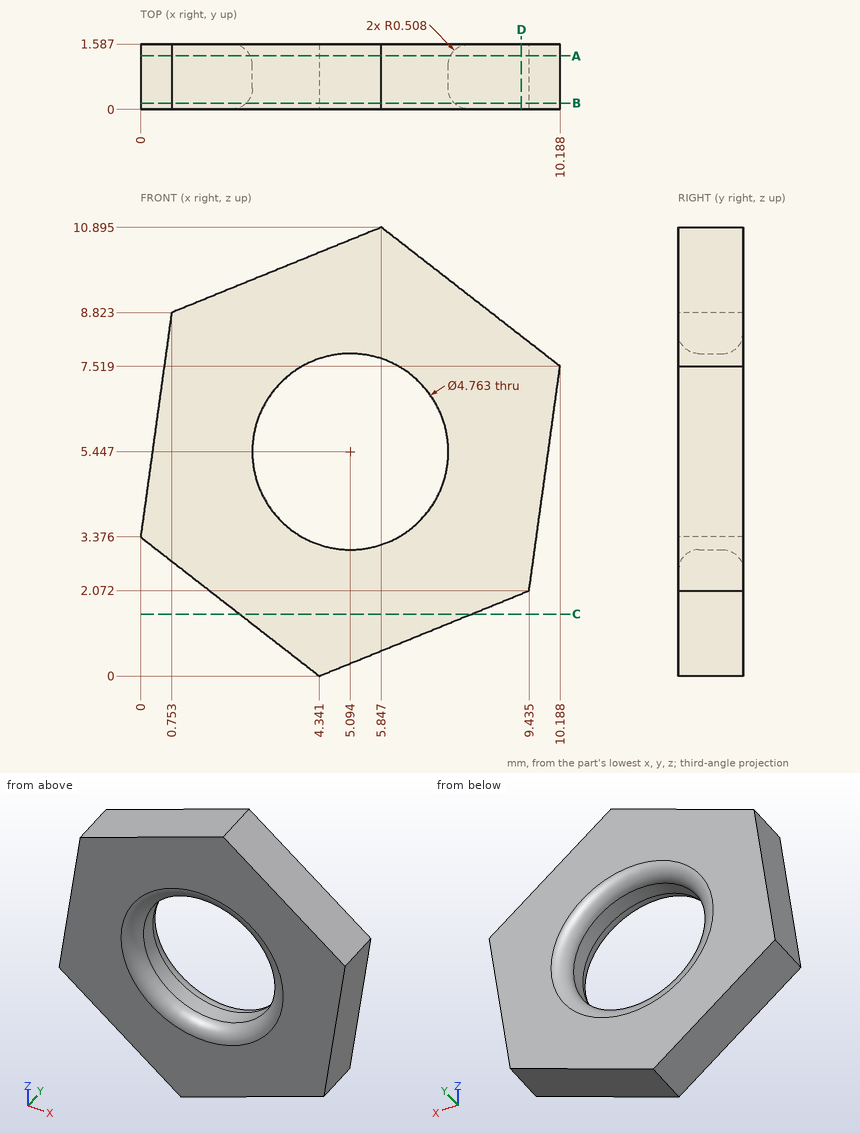
Study the drawing (mm; zero at the part's minimum x, y, z) and answer. Give positions to 0.01 mm unless a question says otherwise; leave off trailing zeros. Loops run counter-clockwise (first coordinate to the right, second up) from the corner with the lowest first, then second, coordinate; pieces in that order, holes last. Notation, with made-up numbers: M -7,-40 L 43,-40 A19 cw 43,-7 Z; hole C 79.25,70.5 d1. An arc over 180 degrees is marked long. Use CSV: the item, a comma, the result in double quotes.
1) Find section B-B on y = 0.15. Write down the section's boundary in (x, z) (1 decimal).
Answer:
outline,"M 0,3.4 L 4.3,0 L 9.4,2.1 L 10.2,7.5 L 5.8,10.9 L 0.8,8.8 Z; hole C 5.1,5.4 d5.1"
2) Find section D-D on x = 9.25. Write down the section's boundary in (y, z).
Answer:
outline,"M 0,2 L 1.59,2 L 1.59,8.25 L 0,8.25 Z"
3) Consider L1, parallel to Z at x = 5.25, y = 0.7 (1 decimal); L2, parallel to Z at x = 4, y = 0.5 (1 decimal); L3, parallel to X at y = 1.45, z = 5.75 (1 decimal). Determine where each line is inside the solid, lowest interval first.
Answer:
L1,"0.4 to 3.1, 7.8 to 10.7"
L2,"0.3 to 3.3, 7.6 to 10.1"
L3,"0.3 to 2.6, 7.6 to 9.9"
4) Find section A-A on y = 1.3. Write down the section's boundary in (x, z) (1 decimal).
Answer:
outline,"M 0,3.4 L 4.3,0 L 9.4,2.1 L 10.2,7.5 L 5.8,10.9 L 0.8,8.8 Z; hole C 5.1,5.4 d4.9"
5) Find section C-C on z = 1.5. Write down the section's boundary in (x, y).
Answer:
outline,"M 2.41,0 L 8.03,0 L 8.03,1.59 L 2.41,1.59 Z"
